Here's the drawing with two shaded views (mm, measured from the low corner). I have some questions. Round coordinates to 2 decimals unless told otherwise and drop trailing zeros. Order: outer loops, then holes, each group sorted by start corner. A loop starts at its lowest first (then second) coordinate and runs counter-clockwise, first axis right, second up.
Q1. If we section it at D-D (x = 23.75): Please give me the cut outline in (y, z).
Q2. If we section it at A-A (y = 11.5): Please give me the cut outline in (x, z).
Q3. Will these pins go through, and if not, where does the flat tip stop? P1, Ø1.2, axis at x = 9, z = 1.5, coming from the -Y side; P2, Ø0.6, axis at x = 10, z = 1.5, coming from the +Y side (1 decimal); P3, Ø1.2, axis at x = 12.5, z = 1.5, coming from the -Y side.
Q4. If we section it at B-B (x = 13): Please give me the cut outline in (y, z).
Q5. If I drill on line 1 (Y direction, x = 12.5, z = 1.8); line 2 (X direction, y = 42.25, z = 1.5); line 3 (Y direction, x = 9, z = 0.5), over which ranges is the centre line in solid material (lowest first)?
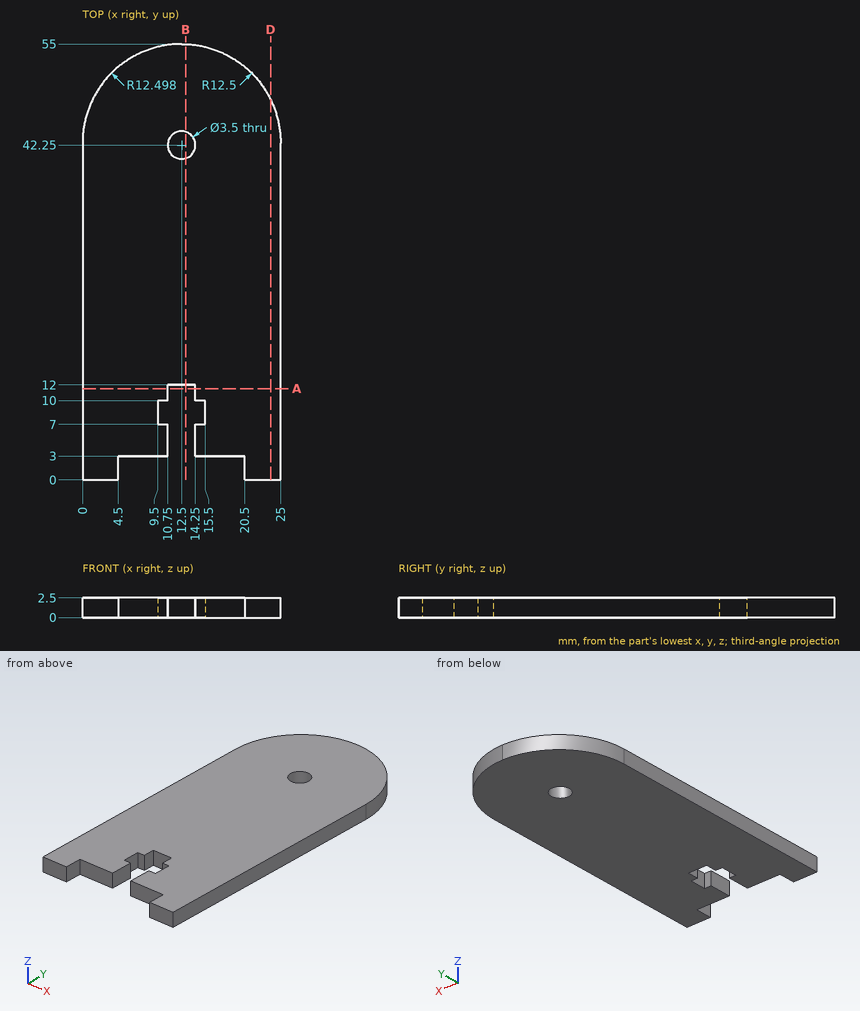
Solution:
1. outline: (0, 0) - (47.95, 0) - (47.95, 2.5) - (0, 2.5) - close
2. outline: (0, 0) - (10.75, 0) - (10.75, 2.5) - (0, 2.5) - close; (14.25, 0) - (25, 0) - (25, 2.5) - (14.25, 2.5) - close
3. P1: stops at y = 3
3. P2: stops at y = 54.8
3. P3: stops at y = 12
4. outline: (12, 0) - (40.57, 0) - (40.57, 2.5) - (12, 2.5) - close; (43.93, 0) - (54.99, 0) - (54.99, 2.5) - (43.93, 2.5) - close
5. line 1: y = 12 to 40.5, 44 to 55
5. line 2: x = 0 to 10.75, 14.25 to 25
5. line 3: y = 3 to 54.5
